Check sheet for the modelled part. Datum: model origin and axes. Units: mm. Face numbers are marked on the shaded views. Give positions to 0.01 mm unless a question says otherwise; leave off trailing zeros. Loops run counter-clockwise (first coordinate to the right, second up) from the corner with the lowest first, then second, coordinate; pieces in that order, holes last. Notation, with made-up numbers: (-18.5, -21) -> (-11.5, -21) arc R14 cw to (-11.5, -3) -> close; hole circle Ø4 at (-12.5, 6). An arc over 180 degrees is marked (long way). Write each question's results on one line, items separated by ' | '. Start each with the question number.
1. Cross-section at A-A on z = 14. Record the boundary of the cut face in (x, y).
2. Mould release check, pull along Y, two halves, no side actions. Record for the marked faces 1, 2, 3 and 4: +Y half, -Y half, draft (parallel to the pull), parting line (faces both ways), or undercut.
3. Cross-section at B-B on z = 8.5. Record the boundary of the cut face in (x, y).
4. Gauge pin test, flat ends, axial feed: pin 1 Ø2 at (y, z) = (-9, 22.5) entering from -X; pin 2 Ø2 at (y, z) = (3.5, 23.5) entering from +X; pin 3 Ø0.6 at (x, z) = (10.5, -4) entering from +Y; pin 4 Ø2 at (y, z) = (-8.5, 2.5) entering from -X. Record the tip position at first contact, or that the pin passes through.
5. Material ranges on L1, parallel to Y at x = 0, z = 12; L2, parallel to Y at x = -3, z = 5.5; L3, parallel to X at y = 9.25, z = 19, recorded low to high. Write a range as from..to.
from build123d import *

# Parameters (mm, degrees)
F0_R      = 10
F1_DEPTH  = 2
F0_R_2    = 12
F2_DEPTH  = 30
F2_FACE_R = 12
F3_DEPTH  = 5
F4_SIZE   = 3
F6_DEPTH  = 16


with BuildPart() as f1:
    # F0 (on Top) → F1 (new body)
    with BuildSketch(Plane.XY):
        Circle(F0_R)
    extrude(amount=F1_DEPTH)

    # F0 (on Top) → F2 (join)
    with BuildSketch(Plane.XY):
        Circle(F0_R_2)
        Circle(F0_R, mode=Mode.SUBTRACT)
    extrude(amount=F2_DEPTH)

    # F2_face (on face) → F3 (join)
    with BuildSketch(Plane(origin=(0, 0, 0), x_dir=(1, 0, 0), z_dir=(0, 0, -1))):
        Circle(F2_FACE_R)
    extrude(amount=F3_DEPTH)

    # F4
    f4_edges = [f1.edges().sort_by_distance(p)[0] for p in [
        (-12, 0, -5),
    ]]
    chamfer(f4_edges, length=F4_SIZE)

    # F5 (on Right) → F6 (join, symmetric)
    with BuildSketch(Plane.YZ):
        with BuildLine():
            Line((0, -4.988678), (0, 28.925132))
            add(Edge.make_bspline(
                [(0, 28.925132), (-1.5119, 29.017054), (-2.72286, 28.264295), (-2.905796, 26.475869)],
                knots=[0, 0, 0, 0, 3.800334, 3.800334, 3.800334, 3.800334], degree=3))
            Line((-2.905796, 26.475869), (-3.372322, 3.091232))
            Line((-3.372322, 3.091232), (-7.718052, -3.04689))
            Line((-7.718052, -3.04689), (-7.718052, -4.988678))
            Line((-7.718052, -4.988678), (0, -4.988678))
        make_face()
        with BuildLine():
            add(Edge.make_bspline(
                [(0, 28.925132), (1.5119, 29.017054), (2.72286, 28.264295), (2.905796, 26.475869)],
                knots=[0, 0, 0, 0, 3.800334, 3.800334, 3.800334, 3.800334], degree=3))
            Line((0, 28.925132), (0, -4.988678))
            Line((0, -4.988678), (7.718052, -4.988678))
            Line((7.718052, -4.988678), (7.718052, -3.04689))
            Line((7.718052, -3.04689), (3.372322, 3.091232))
            Line((3.372322, 3.091232), (2.905796, 26.475869))
        make_face()
    extrude(amount=F6_DEPTH, both=True)


solid = f1.part
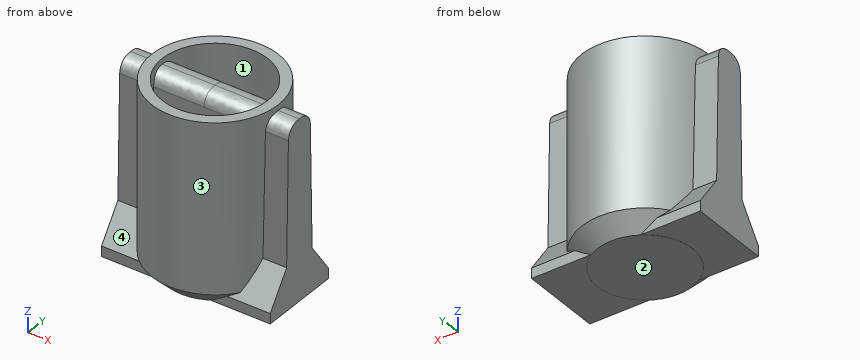
Geometry says:
1) outline: (-16, -3.15) -> (-11.58, -3.15) arc R12 ccw to (11.58, -3.15) -> (16, -3.15) -> (16, 3.15) -> (11.58, 3.15) arc R12 ccw to (-11.58, 3.15) -> (-16, 3.15) -> close; hole (-9.49, -3.15) arc R10 ccw to (9.49, -3.15) -> close; hole (-9.49, 3.15) -> (9.49, 3.15) arc R10 ccw to start
2) face 1: undercut | face 2: draft | face 3: parting line | face 4: -Y half
3) outline: (-16, -3.26) -> (-11.55, -3.26) arc R12 ccw to (11.55, -3.26) -> (16, -3.26) -> (16, 3.26) -> (11.55, 3.26) arc R12 ccw to (-11.55, 3.26) -> (-16, 3.26) -> close; hole (-9.45, -3.26) arc R10 ccw to (9.45, -3.26) -> close; hole (-9.45, 3.26) -> (9.45, 3.26) arc R10 ccw to start
4) pin 1: x = -8.94 | pin 2: x = 16 | pin 3: y = 7.72 | pin 4: x = -9.37
5) L1: -12..-10, -3.19..3.19, 10..12 | L2: -11.62..-9.54, -3.32..3.32, 9.54..11.62 | L3: -7.64..-3.8, 3.8..7.64
